```python
from build123d import *

# Parameters (mm, degrees)
SKETCH1_R             = 4.5
SKETCH1_R_2           = 3.375
BOSS_EXTRUDE1_DEPTH   = 15
CHAMFER1_SIZE         = 0.5
CHAMFER1_SIZE2        = 0.866025404
CHAMFER1_PART_2_SIZE  = 0.5
CHAMFER1_PART_2_SIZE2 = 0.866025404


with BuildPart() as part:
    # Sketch1 → Boss-Extrude1 (new body)
    with BuildSketch(Plane.XY):
        Circle(SKETCH1_R)
        Circle(SKETCH1_R_2, mode=Mode.SUBTRACT)
    extrude(amount=BOSS_EXTRUDE1_DEPTH)

    # Chamfer1
    chamfer1_edges = [part.edges().sort_by_distance(p)[0] for p in [
        (-4.5, 0, 0),
    ]]
    chamfer1_side = [part.faces().sort_by_distance(p)[0] for p in [
        (-4.372720779, 0, 0),
    ]]
    chamfer(chamfer1_edges, length=CHAMFER1_SIZE, length2=CHAMFER1_SIZE2, reference=chamfer1_side[0])

    # Chamfer1 part 2
    chamfer1_part_2_edges = [part.edges().sort_by_distance(p)[0] for p in [
        (-4.5, 0, 15),
    ]]
    chamfer1_part_2_side = [part.faces().sort_by_distance(p)[0] for p in [
        (-4.372720779, 0, 15),
    ]]
    chamfer(chamfer1_part_2_edges, length=CHAMFER1_PART_2_SIZE, length2=CHAMFER1_PART_2_SIZE2, reference=chamfer1_part_2_side[0])


solid = part.part
```
CAD build for the part. Positions are in the model's coordinates, mm. Round coordinates to 2 decimals unless told otherwise and drop trailing zeros. Order: outer loops, then holes, each group sorted by start corner. A loop starts at its lowest first (then second) coordinate and runs counter-clockwise, first axis right, second up. Notation, with made-up numbers: (41.25, -3.75) - (63.25, -3.75) arc R19 ccw to (63.25, 16.25) - close; hole circle Ø11 at (55, -24.5). An arc over 180 degrees is marked (long way). Answer as CSV lines item,"result". Start each with the question number.
1. Pull direction Y, two halves, no side cores. Call faces 1 (the face through (-0.7, -3.3, 7.4)), 2 (the face through (-0.59, 4.46, 7.41)), 3 (the face through (-2, -3, 15)): +Y half, -Y half, draft (parallel to the pull), parting line (faces both ways), or undercut.
2. Saw through at A-A, the plane y = 0. Write the cut outline in (x, z) (3 decimals).
3. Pin check, flat tip, straight feed: pin 1 (1.5 mm diameter, centred on x = 1, y = -1.5, fed in from +Z). Stop position of the tip, or through.
4. Saw through at C-C, the plane z = 8.5. Write the cut outline in (x, y) (3 decimals).
5. Drill centre lines: L1, parallel to Y at x = 0, z = 4.5 (3 decimals); L2, parallel to Y at x = -2, z = 13.25; L3, parallel to X at y = -1, z = 12.5. Where is each one in solid material? Low to high. Write a range as [from, to].
Model answer:
1,face 1,"undercut"
1,face 2,"parting line"
1,face 3,"draft"
2,outline,"(-4.5, 0.866) - (-4, 0) - (-3.375, 0) - (-3.375, 15) - (-4, 15) - (-4.5, 14.134) - close; (3.375, 0) - (4, 0) - (4.5, 0.866) - (4.5, 14.134) - (4, 15) - (3.375, 15) - close"
3,pin 1,"passes through"
4,outline,"circle Ø9 at (0, 0); hole circle Ø6.75 at (0, 0)"
5,L1,"y = [-4.5, -3.375], [3.375, 4.5]"
5,L2,"y = [-4.03, -2.72], [2.72, 4.03]"
5,L3,"x = [-4.39, -3.22], [3.22, 4.39]"
